Input: part model. Units: mm. Frame: model coordinates. Face numbers are marked on the shaded views. A direction names the side the tool comes from. Round coordinates to 2 decimals unless told otherwise and drop trailing zeros. Loops run counter-clockwise (first coordinate to the right, second up) from the corner with the lowest first, then second, coordinate; pieces in that order, holes last.
(1) Access query for the marked faces 5, 6, 7 and 8. Directions: +Z, -Z, +X, -X, +Y, -Y. A direction counts if a zero-diameter tool reaches every point of the face in a straight line with its end or side. Return the directions, or none.
(2) First-contact query: pin 1 Ø3.5 at (y, z) = (33.5, 8) entering from -X; pin 2 Ø4 at (y, z) = (23, 3.5) entering from +X; pin 3 Ø1.6 at (x, z) = (31, 6) entering from -Y; pin 4 Ø1.5 at (y, z) = (10.5, 5) entering from -X. Flat tips, straight axial feed; report the tip coordinate or a pass-through.
(3) Draft query along X for the marked faces 1, 2, 3 and 4. Return one class per face: released by +X, released by -X, zero draft, split by the parting line, or undercut.
(4) Cut plane A-A, the plane z = 7. Output: boundary loops of the cut face in (x, y), and give its area (3 significant figures).
(5) Line query: line 1 (X direction, y = 29, z = 6.75); line 2 (Y direction, x = 53, z = 1); line 3 (Z direction, x = 17, y = 14). Output: solid intervals per line, ascending.
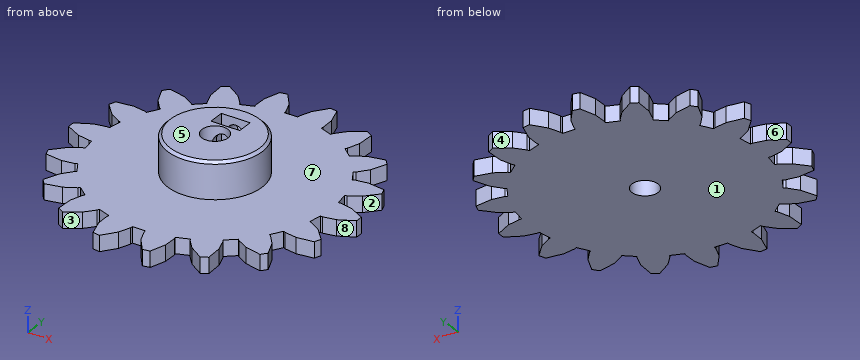
from build123d import *

# Parameters (mm, degrees)
BOSS_EXTRUDE1_DEPTH = 3
SKETCH2_R           = 9
BOSS_EXTRUDE2_DEPTH = 10
SKETCH3_R           = 2.5
CUT_EXTRUDE1_DEPTH  = 11
SKETCH4_R           = 1.7
CUT_EXTRUDE2_DEPTH  = 28.192254919
SKETCH6_W           = 5.5
SKETCH6_H           = 3
CUT_EXTRUDE3_DEPTH  = 6
CHAMFER1_SIZE       = 0.5


with BuildPart() as part:
    # Sketch1 → Boss-Extrude1 (new body)
    with BuildSketch(Plane.XY):
        Polygon((52.538753323, 31.842550454), (52.966828578, 31.892874255), (55.345645602, 31.426138186), (58.181047917, 29.953793943), (58.181047917, 28.58447352), (55.345645602, 27.112129278), (52.966828578, 26.645393209), (52.538753323, 26.695717009), (52.101175487, 24.214740941), (52.520827219, 24.115605549), (54.596406573, 22.863561667), (56.757515266, 20.510014449), (56.289051942, 19.223198182), (53.120822867, 18.809593755), (50.726022805, 19.184537369), (50.340928413, 19.378272292), (49.081325783, 17.196429655), (49.441582758, 16.959930445), (50.963818413, 15.073334341), (52.189727713, 12.122814362), (51.309387982, 11.073577892), (48.190619463, 11.768605458), (46.068603205, 12.939871673), (45.772925049, 13.253692509), (43.84291646, 11.634265293), (44.100798578, 11.288694958), (44.885889814, 8.995405743), (45.028653503, 5.803634881), (43.842700649, 5.118758859), (41.149630401, 6.838401289), (39.556121189, 8.664954435), (39.385711475, 9.061064382), (37.018340862, 8.199298953), (37.142314438, 7.786342725), (37.095662488, 5.362817582), (36.138217708, 2.31467442), (34.789414653, 2.076878813), (32.847095643, 4.613578553), (31.974531237, 6.875118271), (31.949693054, 7.30556898), (29.430487794, 7.30556898), (29.405650376, 6.875118271), (28.53308597, 4.613578553), (26.59076696, 2.076878813), (25.241963905, 2.31467442), (24.284519124, 5.362817582), (24.237867175, 7.786342725), (24.361839986, 8.199298953), (21.994469372, 9.061064382), (21.824060424, 8.664954435), (20.230551212, 6.838401289), (17.537480964, 5.118758859), (16.351527344, 5.803634881), (16.494291033, 8.995405743), (17.279383034, 11.288694958), (17.537264388, 11.634265293), (15.607256564, 13.253692509), (15.311577642, 12.939871673), (13.18956215, 11.768605458), (10.070792865, 11.073577892), (9.190453134, 12.122814362), (10.4163632, 15.073334341), (11.938598855, 16.959930445), (12.29885583, 17.196429655), (11.0392532, 19.378272292), (10.654158042, 19.184537369), (8.259357981, 18.809593755), (5.091129671, 19.223198182), (4.622666347, 20.510014449), (6.783774274, 22.863561667), (8.859354394, 24.115605549), (9.279006126, 24.214740941), (8.841427525, 26.695717009), (8.413353035, 26.645393209), (6.034535245, 27.112129278), (3.199133696, 28.58447352), (3.199133696, 29.953793943), (6.034535245, 31.426138186), (8.413353035, 31.892874255), (8.841427525, 31.842550454), (9.279006126, 34.323526523), (8.859354394, 34.422661915), (6.783774274, 35.674705796), (4.622666347, 38.028253015), (5.091129671, 39.315069282), (8.259357981, 39.728673709), (10.654158042, 39.353730095), (11.0392532, 39.159995172), (12.29885583, 41.341837809), (11.938598855, 41.578337019), (10.4163632, 43.464933122), (9.190453134, 46.415453101), (10.070792865, 47.464689572), (13.18956215, 46.769662005), (15.311577642, 45.598395791), (15.607256564, 45.284574954), (17.537264388, 46.904002171), (17.279383034, 47.249572505), (16.494291033, 49.542861721), (16.351527344, 52.734632582), (17.537480964, 53.419508605), (20.230551212, 51.699866175), (21.824060424, 49.873313028), (21.994469372, 49.477203082), (24.361839986, 50.338968511), (24.237867175, 50.751924739), (24.284519124, 53.175449881), (25.241963905, 56.223593043), (26.59076696, 56.461388651), (28.53308597, 53.92468891), (29.405650376, 51.663149193), (29.430487794, 51.232698484), (31.949693054, 51.232698484), (31.974531237, 51.663149193), (32.847095643, 53.92468891), (34.789414653, 56.461388651), (36.138217708, 56.223593043), (37.095662488, 53.175449881), (37.142314438, 50.751924739), (37.018340862, 50.338968511), (39.385711475, 49.477203082), (39.556121189, 49.873313028), (41.149630401, 51.699866175), (43.842700649, 53.419508605), (45.028653503, 52.734632582), (44.885889814, 49.542861721), (44.100798578, 47.249572505), (43.84291646, 46.904002171), (45.772925049, 45.284574954), (46.068603205, 45.598395791), (48.190619463, 46.769662005), (51.309387982, 47.464689572), (52.189727713, 46.415453101), (50.963818413, 43.464933122), (49.441582758, 41.578337019), (49.081325783, 41.341837809), (50.340928413, 39.159995172), (50.726022805, 39.353730095), (53.120822867, 39.728673709), (56.289051942, 39.315069282), (56.757515266, 38.028253015), (54.596406573, 35.674705796), (52.520827219, 34.422661915), (52.101175487, 34.323526523), align=None)
    extrude(amount=BOSS_EXTRUDE1_DEPTH)

    # Sketch2 → Boss-Extrude2 (add)
    with BuildSketch(Plane.XY):
        with Locations((30.690090806, 29.269133732)):
            Circle(SKETCH2_R)
    extrude(amount=BOSS_EXTRUDE2_DEPTH)

    # Sketch3 → Cut-Extrude1 (cut, through all)
    with BuildSketch(Plane.XY):
        with Locations((30.690090424, 29.269133732)):
            Circle(SKETCH3_R)
    extrude(amount=CUT_EXTRUDE1_DEPTH, mode=Mode.SUBTRACT)

    # Sketch4 → Cut-Extrude2 (cut, through all)
    with BuildSketch(Plane(origin=(0, 29.269133732, 0), x_dir=(1, 0, 0), z_dir=(0, 1, 0))):
        with Locations((30.690090424, -7)):
            Circle(SKETCH4_R)
    extrude(amount=CUT_EXTRUDE2_DEPTH, mode=Mode.SUBTRACT)

    # Sketch6 → Cut-Extrude3 (cut)
    with BuildSketch(Plane.XY.offset(10)):
        with Locations((30.690090806, 33.769133732)):
            Rectangle(SKETCH6_W, SKETCH6_H)
    extrude(amount=-CUT_EXTRUDE3_DEPTH, mode=Mode.SUBTRACT)

    # Chamfer1
    chamfer1_edges = [part.edges().sort_by_distance(p)[0] for p in [
        (21.690090806, 29.269133732, 10),
    ]]
    chamfer(chamfer1_edges, length=CHAMFER1_SIZE)


solid = part.part
Reported:
1. face 5: +Z, +X, -X, +Y, -Y
1. face 6: +Z, -Z, -X
1. face 7: +Z
1. face 8: +Z, -Z, +X
2. pin 1: stops at x = 22.04
2. pin 2: stops at x = 56.25
2. pin 3: stops at y = 20.27
2. pin 4: passes through
3. face 1: zero draft
3. face 2: released by +X
3. face 3: undercut
3. face 4: undercut
4. outline: (27.94, 32.27) - (27.94, 35.27) - (28.99, 35.27) - (28.99, 38.11) arc R9 ccw (long way) to (32.39, 38.11) - (32.39, 35.27) - (33.44, 35.27) - (33.44, 32.27) - (32.39, 32.27) - (32.39, 31.1) arc R2.5 cw (long way) to (28.99, 31.1) - (28.99, 32.27) - close
4. area: 206 mm2
5. line 1: x = 21.69 to 28.2, 33.18 to 39.69
5. line 2: y = 18.83 to 23.83, 26.65 to 31.89, 34.71 to 39.71
5. line 3: z = 0 to 3
